Geometry: see drawing. Coordinates: mm, zero at the bounding-box minimum. A direction names the side the tool comes from. Give positions to 0.01 mm unless a question says otherwise; leave off trailing zeros. Order: outer loops, then holes, each group sorted by start corner. A loop starts at its lowest first (then second) coordinate and runs counter-clockwise, first axis right, second up. Notation, with made-up numbers: (14, 84.5) - (44, 84.5) arc R21 cw to (44, 89.5) - close; hole circle Ø7 at (43, 38.25). An arc over 180 degrees is marked (long way). Put each result on its own line as item: value. Start each with the question number.
1. Section A-A on z = 5. Return the cut outline in (x, y), plus the area to 3 significant figures.
2. Mould query, pull axis Y, two halves, no side actions, for the marked faces 1, 2 and 3. Classes: pulls with the +Y half, pulls with the -Y half, needs draft (parallel to the pull), parting line crosses it, or undercut.
3. Set-up query: the marked faces 4, 5 and 6. Return all of +Z, -Z, +X, -X, +Y, -Y with unobstructed straight access to the full face (end or side cutting, diameter ignored); none if empty.
4. Ray query, line 1 along Y through (x, z) = (5.09, 16.65); line 2 along Z through (x, y) = (36.5, 1.7); line 3 along X through (y, z) = (2.95, 35). Return the intervals inside material, ascending. Write a range as from..to.
5. Section B-B on x = 36.5. Return the cut outline in (y, z).
6. Section D-D on x = 5.09. Count the separate pieces of the cut face and the enclosed holes in it, plus the area to 3 significant figures.
7. First-contact query: P1, Ø5, axis at x = 5.09, y = 48.67, coming from the -Z side; P2, Ø5, axis at x = 16, z = 17, coming from the -Y side; P3, Ø4, axis at y = 22.5, z = 15.5, coming from the -X side; P4, Ø1.5, axis at y = 2, z = 13.5, coming from the -X side. Flat tips, straight axial feed; report the tip coordinate or a pass-through.
8. Section C-C on z = 17. Return the cut outline in (x, y).
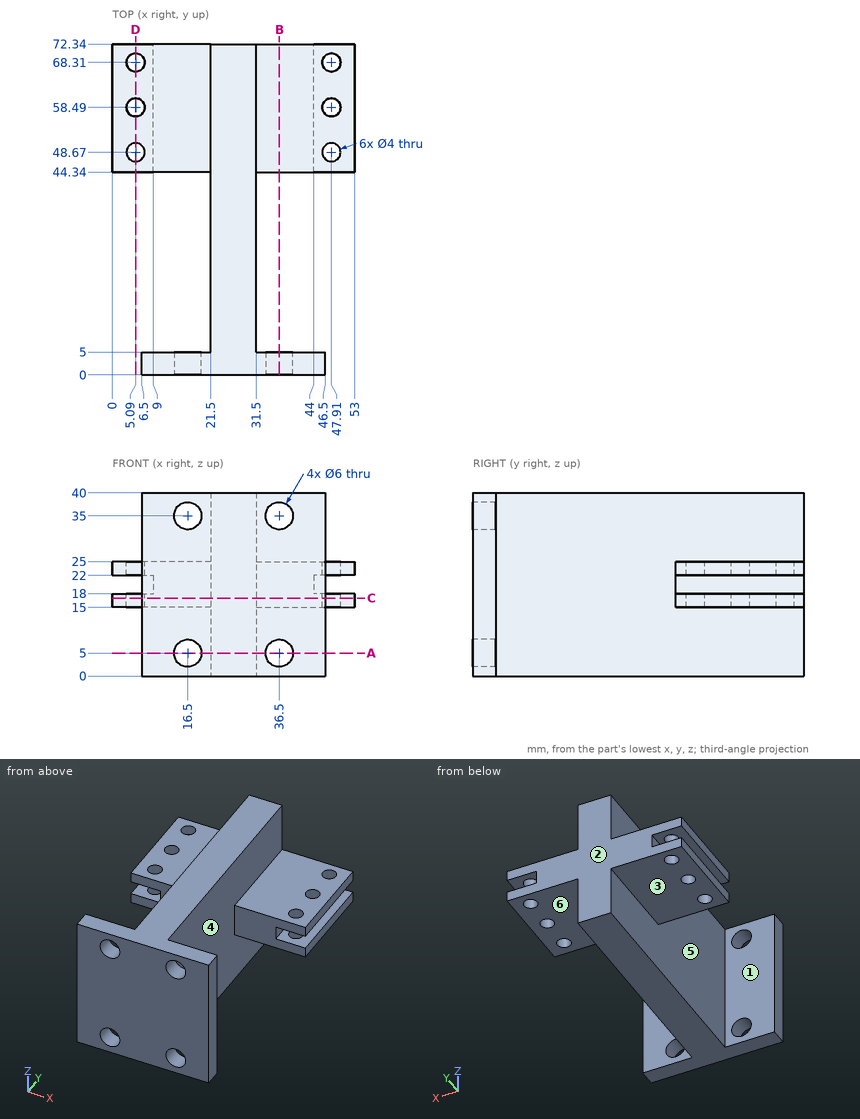
Resolved:
1. outline: (6.5, 0) - (13.5, 0) - (13.5, 5) - (6.5, 5) - close; (19.5, 0) - (33.5, 0) - (33.5, 5) - (31.5, 5) - (31.5, 72.34) - (21.5, 72.34) - (21.5, 5) - (19.5, 5) - close; (39.5, 0) - (46.5, 0) - (46.5, 5) - (39.5, 5) - close
1. area: 813 mm^2
2. face 1: undercut
2. face 2: pulls with the +Y half
2. face 3: needs draft
3. face 4: +X
3. face 5: -X
3. face 6: -Z, +X, +Y
4. line 1: 44.34..46.67, 50.67..56.49, 60.49..66.31, 70.31..72.34
4. line 2: 0..2, 8..32, 38..40
4. line 3: 6.5..13.5, 19.5..33.5, 39.5..46.5
5. outline: (0, 0) - (5, 0) - (5, 2) - (0, 2) - close; (0, 8) - (5, 8) - (5, 32) - (0, 32) - close; (0, 38) - (5, 38) - (5, 40) - (0, 40) - close; (44.34, 15) - (72.34, 15) - (72.34, 25) - (44.34, 25) - close
6. separate pieces: 8
6. enclosed holes: 0
6. area: 96.0 mm^2
7. P1: z = 15
7. P2: y = 0
7. P3: x = 21.5
7. P4: x = 6.5
8. outline: (0, 44.34) - (21.5, 44.34) - (21.5, 5) - (6.5, 5) - (6.5, 0) - (46.5, 0) - (46.5, 5) - (31.5, 5) - (31.5, 44.34) - (53, 44.34) - (53, 72.34) - (0, 72.34) - close; hole circle Ø4 at (5.09, 48.67); hole circle Ø4 at (5.09, 58.49); hole circle Ø4 at (5.09, 68.31); hole circle Ø4 at (47.91, 48.67); hole circle Ø4 at (47.91, 58.49); hole circle Ø4 at (47.91, 68.31)
